Input: part model. Units: mm. Frame: model coordinates. A direction names the side the tool comes from. Coordinates: 2 decimals unless noted, no trailing zeros. Write each loop counter-clockwise with the first axis right and the second up, starting at its lowest first coordinate (ties: lowest second). Pieces come first, ordered by that corner, then holes. Notation, with made-up numbers: M -2.75,-23 L 13.25,-23 A27 cw 13.25,3 Z; hole C 48.5,-32 d5. An arc over 180 degrees is marked long. Answer as a JSON object with one key per item and string values. Group by question number.
from build123d import *

# Parameters (mm, degrees)
SKETCH1_W                    = 50
SKETCH1_H                    = 40
BASE_FLANGE1_DEPTH           = 2
EDGE_FLANGE1_STRIP_W         = 9.4732
EDGE_FLANGE1_STRIP_H         = 2
EDGE_FLANGE1_STRIP_CUT_DEPTH = 40
EDGE_FLANGE1_DEPTH           = 40
SKETCH14_R                   = 4
CUT_EXTRUDE2_DEPTH           = 10
FILLET1_R                    = 2
FILLET1_OF_MIRROR2_R         = 2
SKETCH23_R                   = 10
CUT_EXTRUDE3_DEPTH           = 10


# Sheet-metal steps are written as plain solids
with BuildPart() as part:
    # Sketch1 → Base-Flange1 (new body)
    with BuildSketch(Plane(origin=(0, 0, 0), x_dir=(1, 0, 0), z_dir=(0, 1, 0))):
        Rectangle(SKETCH1_W, SKETCH1_H)
    extrude(amount=-BASE_FLANGE1_DEPTH)

    # Edge-Flange1 strip (across the edge) → Edge-Flange1 strip cut (cut)
    with BuildSketch(Plane(origin=(-25, 0, -20), x_dir=(1, 0, 0), z_dir=(0, 0, 1))):
        with Locations((-2, -1)):
            Rectangle(EDGE_FLANGE1_STRIP_W, EDGE_FLANGE1_STRIP_H)
    edge_flange1_strip_cut = extrude(amount=EDGE_FLANGE1_STRIP_CUT_DEPTH, mode=Mode.SUBTRACT)

    # Edge-Flange1 section (across the edge) → Edge-Flange1 (add)
    with BuildSketch(Plane(origin=(-25, 0, -20), x_dir=(1, 0, 0), z_dir=(0, 0, 1))):
        with BuildLine():
            Line((0, 0.7366), (0, 36))
            Line((0, 36), (2, 36))
            Line((2, 36), (2, 0.7366))
            ThreePointArc((2, 0.7366), (2.215745145, 0.215745145), (2.7366, 0))
            Line((2.7366, 0), (2.7366, -2))
            ThreePointArc((2.7366, -2), (0.801531583, -1.198468417), (0, 0.7366))
        make_face()
    edge_flange1 = extrude(amount=EDGE_FLANGE1_DEPTH)

    # Sketch14 → Cut-Extrude2 (cut)
    with BuildSketch(Plane.ZY.offset(25)):
        with BuildLine():
            Line((-20, 0.7366), (-7.38689697, 31.071441544))
            ThreePointArc((-7.38689697, 31.071441544), (-4.440071376, 34.654755155), (0, 36))
            Line((0, 36), (-20, 36))
            Line((-20, 36), (-20, 0.7366))
        make_face()
        with BuildLine():
            Line((20, 36), (0, 36))
            ThreePointArc((0, 36), (4.440071376, 34.654755155), (7.38689697, 31.071441544))
            Line((7.38689697, 31.071441544), (20, 0.7366))
            Line((20, 0.7366), (20, 36))
        make_face()
        with BuildLine():
            Line((-5.608456521, 19.720796207), (-12.145099279, 4))
            Line((-12.145099279, 4), (12.145099279, 4))
            Line((12.145099279, 4), (5.608456521, 19.720796207))
            ThreePointArc((5.608456521, 19.720796207), (0, 18), (-5.608456521, 19.720796207))
        make_face()
        with Locations(Location((0, 28, 0), (0, 0, 270))):
            Circle(SKETCH14_R)
    cut_extrude2 = extrude(amount=-CUT_EXTRUDE2_DEPTH, mode=Mode.SUBTRACT)

    # Fillet1
    fillet1_edges = [part.edges().sort_by_distance(p)[0] for p in [
        (-24, 19.720796207, -5.608456521),
        (-24, 19.720796207, 5.608456521),
        (-24, 4, 12.145099279),
        (-24, 4, -12.145099279),
    ]]
    fillet(fillet1_edges, radius=FILLET1_R)

    # Mirror2: Edge-Flange1 strip cut, Edge-Flange1, Cut-Extrude2 across plane
    add(edge_flange1_strip_cut.mirror(Plane(origin=(0, 0, 0), x_dir=(0, 0, 1), z_dir=(1, 0, 0))), mode=Mode.SUBTRACT)
    add(edge_flange1.mirror(Plane(origin=(0, 0, 0), x_dir=(0, 0, 1), z_dir=(1, 0, 0))))
    add(cut_extrude2.mirror(Plane(origin=(0, 0, 0), x_dir=(0, 0, 1), z_dir=(1, 0, 0))), mode=Mode.SUBTRACT)

    # Fillet1 of Mirror2
    fillet1_of_mirror2_edges = [part.edges().sort_by_distance(p)[0] for p in [
        (24, 19.720796207, -5.608456521),
        (24, 19.720796207, 5.608456521),
        (24, 4, 12.145099279),
        (24, 4, -12.145099279),
    ]]
    fillet(fillet1_of_mirror2_edges, radius=FILLET1_OF_MIRROR2_R)

    # Sketch23 → Cut-Extrude3 (cut)
    with BuildSketch(Plane(origin=(0, 0, 0), x_dir=(1, 0, 0), z_dir=(0, 1, 0))):
        with Locations(Location((0, 0, 0), (0, 0, 270))):
            Circle(SKETCH23_R)
    extrude(amount=-CUT_EXTRUDE3_DEPTH, mode=Mode.SUBTRACT)


solid = part.part
Q1. Access query for faces 5 (the flat face through (-23, 19, 0)), 6 (the flat face through (-25, 22, 0)), 7 (the flat face through (24.014, 12.304, -8.692)). Directions: +Z, -Z, +X, -X, +Y, -Y. A direction counts if a zero-diameter tool reaches every point of the face in a straight line with its end or side. Return the directions, or none.
Q2. Section B-B, the plane y = 29. Return the cut outline in (x, z).
Q3. Section D-D, the plane y = 8. Return the cut outline in (x, z).
Q4. Section C-C, the plane z = 1.5. State how many separate pieces and enclosed holes the cut face has, and give its area (3 significant figures).
Q5. Line query: line 1 (X direction, y = 17, z = -10); line 2 (Y direction, x = 23.6, z = 0); line 3 (Y direction, x = 24, z = 0). Output: solid intervals per line, ascending. Write a range as from..to.
Q6. Draft query along Y for faces 1 (the flat face through (-24.014, 16.116, 13.605)), 2 (the flat face through (0, -1, -20)), 3 (the cylindrical face through (24.177, -1.22, -0.28)), 4 (the cylindrical face through (23.986, 4.913, -10.826)). Return one class per face: released by +Y, released by -Y, zero draft, split by the parting line, or undercut.
Q7. Section A-A, the plane x = 0. Return the cut outline in (y, z), and give its area (3 significant figures).
Q8. Pin query (flat end, axial travel): pin 1 Ø10 at (x, z) = (5.5, -1.5) entering from +Y; pin 2 Ø5 at (y, z) = (15.5, -2.5) entering from -X; pin 3 Ø1.6 at (x, z) = (24, 1.5) entering from +Y. Return the tip coordinate at first contact, or that it passes through.
Filled in:
{
 "1": {"face 5": "+Z, -Z, +Y", "face 6": "+Z, -Z, -X, +Y, -Y", "face 7": "+X, -X"},
 "2": {"outline": "M -25,-8.25 L -23,-8.25 L -23,-3.87 L -25,-3.87 Z; M -25,3.87 L -23,3.87 L -23,8.25 L -25,8.25 Z; M 23,-8.25 L 25,-8.25 L 25,-3.87 L 23,-3.87 Z; M 23,3.87 L 25,3.87 L 25,8.25 L 23,8.25 Z"},
 "3": {"outline": "M -25,-16.98 L -23,-16.98 L -23,-10.48 L -25,-10.48 Z; M -25,10.48 L -23,10.48 L -23,16.98 L -25,16.98 Z; M 23,-16.98 L 25,-16.98 L 25,-10.48 L 23,-10.48 Z; M 23,10.48 L 25,10.48 L 25,16.98 L 23,16.98 Z"},
 "4": {"separate pieces": "6", "enclosed holes": "0", "area": "115 mm^2"},
 "5": {"line 1": "-25..-23, 23..25", "line 2": "-1.65..4, 18..24, 32..36", "line 3": "-1.38..4, 18..24, 32..36"},
 "6": {"face 1": "released by +Y", "face 2": "zero draft", "face 3": "released by -Y", "face 4": "undercut"},
 "7": {"outline": "M -2,-20 L 0,-20 L 0,-10 L -2,-10 Z; M -2,10 L 0,10 L 0,20 L -2,20 Z", "area": "40.0 mm^2"},
 "8": {"pin 1": "y = 0", "pin 2": "through", "pin 3": "y = 35.97"}
}
